Here's how the part is built. I have some questions about the finished solid (model axes, mm). A direction names the side the tool comes from. Coordinates: 2 decimals unless noted, no trailing zeros. Write each loop counter-clockwise with the first axis right and the second up, starting at its lowest first coordinate (ties: lowest second). Pieces come first, ordered by that corner, then holes.
(1) Imagine slicing it at B-B, the plane x = 0. List the corners of the cut face in (y, z) for me.
(2) Imagine slicing it at C-C, the plane y = -6.5. List the corners of the cut face in (x, z) for me, plus the area to 3 significant figures.
(3) Thinking about a two-plate mould opening in X: for faces 4 (the cylindrical face through (5.173, -292.054, 1.07)), 5 (the flat face through (163, -79, -76.2)), 6 (the flat face through (-44.45, 77, 1)), 7 (the cylindrical face through (-4.13, 229.053, 1.07)), which applies, released by +X, released by -X, zero draft, split by the parting line, or undercut?
(4) Please list where these lines run through material, in increasing order: probe 1 along Z at (x, y) = (188, -129.5); probe 2 along X at (y, z) = (247, -25); probe 3 along X at (y, z) = (239.5, -28).
(5) Which directions (+Z, -Z, +X, -X, +Y, -Y) give clear straight access to the entire face, cutting with the end or side of a thin tool? Please do faces 1 (the flat face through (4, -126, 76.454)), 2 (the flat face through (163, -79, 76.2)), 3 (the flat face through (-160, -79, -76.2)).
(6) For pin 1 Ø3 at (x, z) = (36.5, -27.5) entering from -Y; pin 2 Ø6 at (x, z) = (107, 46) entering from +Y; pin 3 Ø2 at (x, z) = (160, 58) entering from +Y, each with a flat end and sliding along its axis, tell me the tip position at first contact or that it passes through.
(7) Imagine slicing it at D-D, the plane x = 195. List the corners of the cut face in (y, z) for me.
(8) Imagine slicing it at A-A, the plane z = 56. List the corners of the cut face in (x, y) for me, plus the area to 3 significant figures.
```python
from build123d import *

# Parameters (mm, degrees)
SKETCH1_R           = 19.05
BOSS_EXTRUDE2_DEPTH = 76.2
SKETCH3_R           = 12.7
SKETCH3_R_2         = 19.05
BOSS_EXTRUDE4_DEPTH = 0.254


with BuildPart() as part:
    # Sketch1 → Boss-Extrude2 (new body, symmetric)
    with BuildSketch(Plane.XY):
        with BuildLine():
            Line((-44.45, -88.9), (-238.151556269, -169.13381166))
            ThreePointArc((-238.151556269, -169.13381166), (0, -292.1), (238.151556269, -169.13381166))
            Line((238.151556269, -169.13381166), (44.45, -88.9))
            Line((44.45, -88.9), (44.45, 247.65))
            ThreePointArc((44.45, 247.65), (0, 292.1), (-44.45, 247.65))
            Line((-44.45, 247.65), (-44.45, -88.9))
        make_face()
        with Locations((0, 247.65)):
            Circle(SKETCH1_R, mode=Mode.SUBTRACT)
    extrude(amount=BOSS_EXTRUDE2_DEPTH, both=True)

    # Sketch3 → Boss-Extrude4 (add)
    with BuildSketch(Plane.XY.offset(76.2)):
        with BuildLine():
            Line((44.45, 247.65), (44.45, 9.08096904))
            Line((44.45, 9.08096904), (278.563150245, -87.891872921))
            ThreePointArc((278.563150245, -87.891872921), (0, -292.1), (-278.563150245, -87.891872921))
            Line((-278.563150245, -87.891872921), (-44.45, 9.08096904))
            Line((-44.45, 9.08096904), (-44.45, 247.65))
            ThreePointArc((-44.45, 247.65), (0, 292.1), (44.45, 247.65))
        make_face()
        with Locations((-117.332700629, -48.60079591)):
            Circle(SKETCH3_R, mode=Mode.SUBTRACT)
        with Locations((117.332700629, -48.60079591)):
            Circle(SKETCH3_R, mode=Mode.SUBTRACT)
        with Locations((0, 247.65)):
            Circle(SKETCH3_R_2, mode=Mode.SUBTRACT)
    boss_extrude4 = extrude(amount=BOSS_EXTRUDE4_DEPTH)

    # Mirror4: Boss-Extrude4 across plane
    add(boss_extrude4.mirror(Plane.XY))


solid = part.part
```
Recorded:
1. outline: (-292.1, -76.45) - (228.6, -76.45) - (228.6, 76.45) - (-292.1, 76.45) - close; (266.7, -76.45) - (292.1, -76.45) - (292.1, 76.45) - (266.7, 76.45) - close
2. outline: (-82.07, -76.45) - (82.07, -76.45) - (82.07, -76.2) - (44.45, -76.2) - (44.45, 76.2) - (82.07, 76.2) - (82.07, 76.45) - (-82.07, 76.45) - (-82.07, 76.2) - (-44.45, 76.2) - (-44.45, -76.2) - (-82.07, -76.2) - close
2. area: 13,600 mm2
3. face 4: split by the parting line
3. face 5: zero draft
3. face 6: released by -X
3. face 7: undercut
4. probe 1: z = -76.45 to -76.2, 76.2 to 76.45
4. probe 2: x = -44.45 to -19.04, 19.04 to 44.45
4. probe 3: x = -44.45 to -17.22, 17.22 to 44.45
5. face 1: +Z, +X, -X, +Y, -Y
5. face 2: +X, +Y
5. face 3: -X, +Y
6. pin 1: stops at y = -290
6. pin 2: stops at y = -113.57
6. pin 3: stops at y = -136.35
7. outline: (-217.48, -76.45) - (-53.28, -76.45) - (-53.28, -76.2) - (-151.26, -76.2) - (-151.26, 76.2) - (-53.28, 76.2) - (-53.28, 76.45) - (-217.48, 76.45) - close
8. outline: (-238.15, -169.13) arc R292.1 ccw to (238.15, -169.13) - (44.45, -88.9) - (44.45, 247.65) arc R44.45 ccw to (-44.45, 247.65) - (-44.45, -88.9) - close; hole circle Ø38.1 at (0, 247.65)
8. area: 95,600 mm2
